Input: dimensioned drawing with shaded views. Units: mm. Origin: part minimum x, y, z. A direction names the side the tool comes from. Coordinates: 2 decimals unless noted, no trailing zeros. Order: outer loops, then holes, each group sorted by start corner. A loop starts at its lowest first (then second) coordinate and runs counter-clockwise, first axis right, second up.
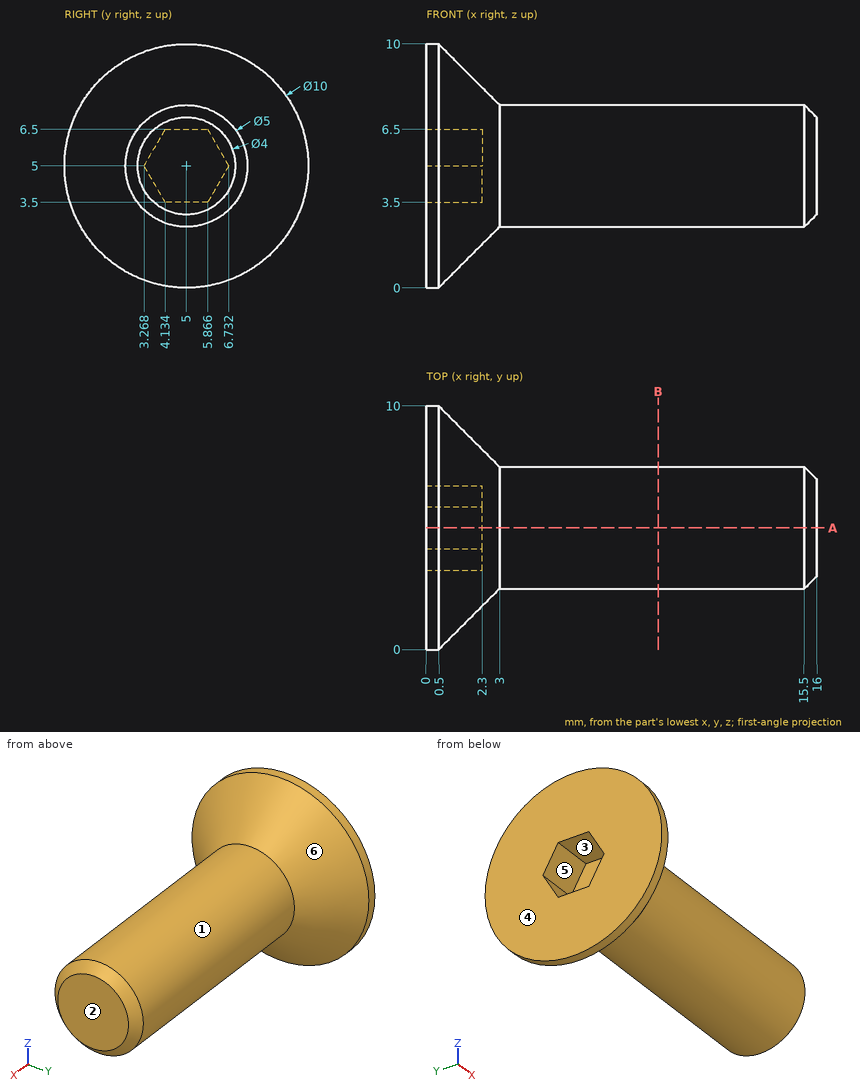
1. Section query A-A on y = 5. Return loops of the section in (x, z), plus the area to 3 significant figures.
Findings:
outline: (0, 0) - (0.5, 0) - (3, 2.5) - (15.5, 2.5) - (16, 3) - (16, 7) - (15.5, 7.5) - (3, 7.5) - (0.5, 10) - (0, 10) - (0, 6.5) - (2.3, 6.5) - (2.3, 3.5) - (0, 3.5) - close
area: 81.6 mm2
2. Access query for the marked faces 1, 2 and 3. Directions: +Z, -Z, +X, -X, +Y, -Y. A direction counts if a zero-diameter tool reaches every point of the face in a straight line with its end or side. Return the directions, or none.
Findings:
face 1: +X
face 2: +Z, -Z, +X, +Y, -Y
face 3: -X
3. Section query B-B on x = 9.5. Return loops of the section in (y, z), plus the area to 3 significant figures.
Findings:
outline: circle Ø5 at (5, 5)
area: 19.6 mm2
4. Pin query (flat end, axial travel): P1, Ø1.9, axis at x = 1.5, y = 5, coming from the -Z side; P2, Ø1.5, axis at y = 3.5, z = 2, coming from the +X side; P3, Ø1.9, axis at x = 1.5, y = 5, coming from the +Z side. Return the tip coordinate at first contact, or that it passes through.
Findings:
P1: stops at z = 0.05
P2: stops at x = 2.9
P3: stops at z = 9.95
5. Ray query, line 1 (Y direction, x = 12, z = 6.5); line 2 (Z direction, x = 7.25, y = 5); line 3 (X direction, y = 5.5, z = 4.5). Return the intervals inside material, ascending.
Findings:
line 1: y = 3 to 7
line 2: z = 2.5 to 7.5
line 3: x = 2.3 to 16
6. Draft query along Z for the marked faces 4, 5 and 6. Return one class per face: released by +Z, released by -Z, zero draft, split by the parting line, or undercut.
Findings:
face 4: zero draft
face 5: undercut
face 6: split by the parting line
